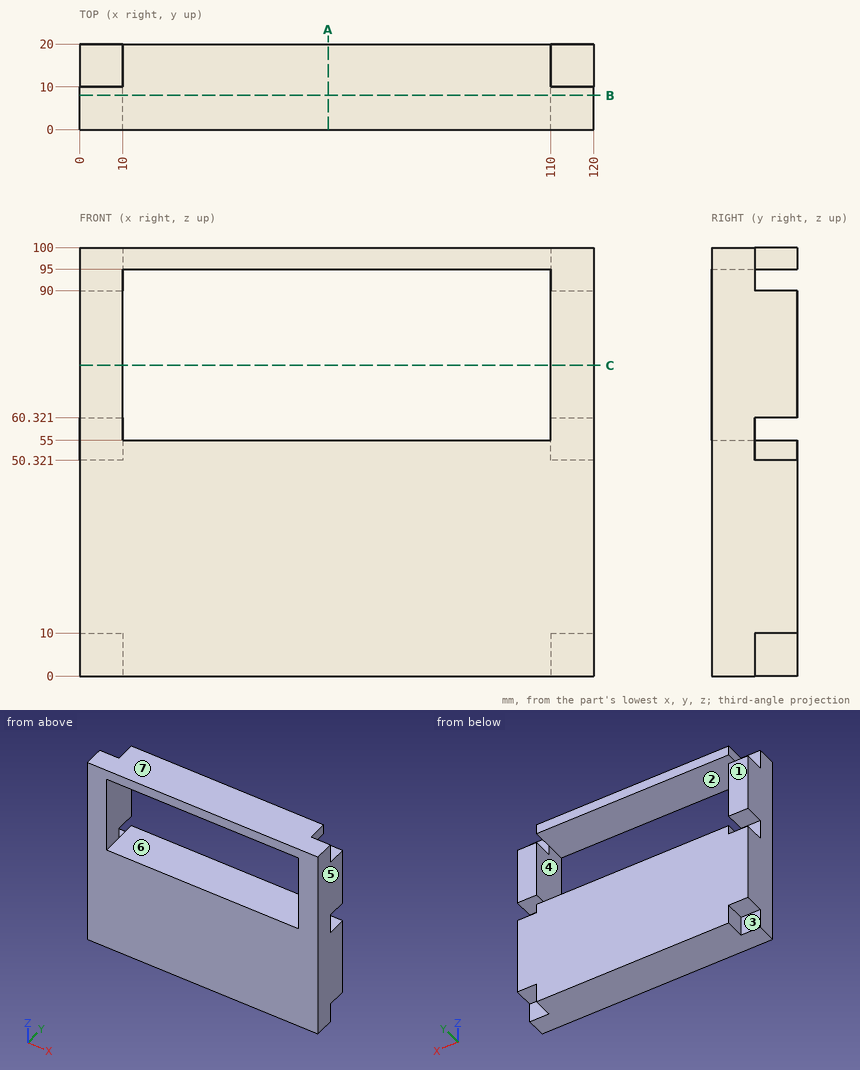
Print and shaded views of the part. All mm, measured from the part's lowest x, y and z. A direction names the side the tool comes from. Coordinates: 2 decimals unless noted, no trailing zeros. Order: outer loops, then holes, each group sorted by start corner. A loop starts at its lowest first (then second) coordinate and runs counter-clockwise, first axis right, second up. Notation, with made-up numbers: (-30, 19) - (1, 19) arc R33 cw to (1, 54) - close; hole circle Ø7 at (18.25, 46). An arc over 180 degrees is marked (long way). Return JSON: item names as keys, results as strings. Group by question number.
Item 1: Which spindle directions (+Z, -Z, +X, -X, +Y, -Y) get a long thin tool onto all of the face, cutting with end or side? Do the marked faces 1, 2 and 3. Say none if no direction does.
Item 2: Cut at B-B (y = 8). List the corners of the cut face in (x, z), plus the area to 3 significant figures.
Item 3: Drill centre lines: probe 1 along Z at (x, y) = (109, 7.5); probe 2 along X at (y, z) = (3, 73.5); probe 3 along Z at (x, y) = (114, 17.25). Where is each one in solid material? Low to high. Write a range as from..to.
Item 4: Cut at A-A (x = 58). List the corners of the cut face in (y, z).
Item 5: Pin check, flat tips, straight feed: pin 1 (11 mm diameter, centred on x = 117, y = 13.5, fed in from +Z); pin 2 (5 mm diameter, centred on x = 116.5, z = 57.5, fed in from +Y); pin 3 (5 mm diameter, centred on x = 3, y = 16, fed in from +Z); pin 4 (3 mm diameter, centred on x = 115, y = 12.5, fed in from -Z). Stop position of each tip, or through.
Item 6: Cut at C-C (z = 72.5). List the corners of the cut face in (x, y).
Item 7: Pull direction X, two halves, no side cores. Call the marked faces 4, 5, 6 and 7: pulls with the +X half, pulls with the -X half, needs draft (parallel to the pull), parting line crosses it, or undercut.
Check values:
{
 "1": {"face 1": "+Z, -Z, +X, -X, +Y", "face 2": "+Y, -Y", "face 3": "-Z, -X, +Y"},
 "2": {"outline": "(0, 0) - (120, 0) - (120, 100) - (0, 100) - close; hole (10, 55) - (110, 55) - (110, 95) - (10, 95) - close", "area": "8,000 mm2"},
 "3": {"probe 1": "z = 0..55, 95..100", "probe 2": "x = 0..10, 110..120", "probe 3": "z = 10..50.32, 60.32..90"},
 "4": {"outline": "(0, 0) - (20, 0) - (20, 55) - (0, 55) - close; (0, 95) - (20, 95) - (20, 100) - (0, 100) - close"},
 "5": {"pin 1": "stops at z = 100", "pin 2": "stops at y = 10", "pin 3": "stops at z = 90", "pin 4": "stops at z = 10"},
 "6": {"outline": "(0, 0) - (10, 0) - (10, 20) - (0, 20) - close; (110, 0) - (120, 0) - (120, 20) - (110, 20) - close"},
 "7": {"face 4": "undercut", "face 5": "pulls with the +X half", "face 6": "undercut", "face 7": "needs draft"}
}
